Source: CAD feature listing. Evaluate the final solid. Frame: model axes, mm. Give positions to 0.01 mm unless a question says otherwise; leave off trailing zeros. Loops run counter-clockwise (first coordinate to the right, second up) from the corner with the lowest first, then second, coordinate; pieces in that order, holes last. Notation, with made-up numbers: (5.25, -20) - (39.25, -20) arc R24 cw to (39.25, 4) - close; hole circle Ø7 at (-25.5, 79). An arc over 180 degrees is marked (long way). Put each result on its own line as item: value.
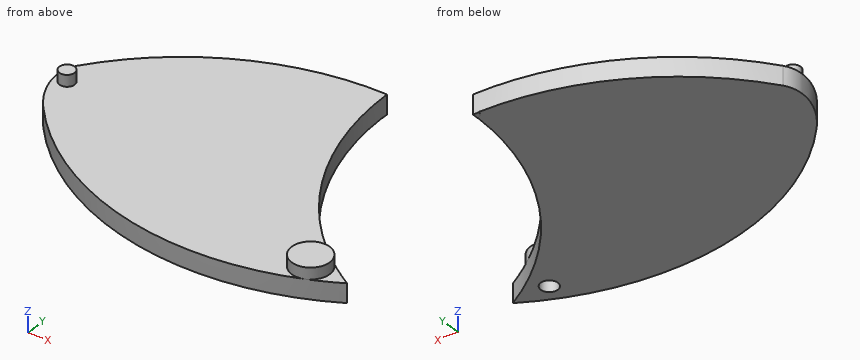
```python
from build123d import *

# Parameters (mm, degrees)
ESTRUSIONE_ESTRUSIONE1_DEPTH = 5
SCHIZZO2_R                   = 2
ESTRUSIONE_ESTRUSIONE3_DEPTH = 3
SCHIZZO3_R                   = 2.25
TAGLIO_ESTRUSIONE2_DEPTH     = 5
SCHIZZO4_R                   = 5
ESTRUSIONE_ESTRUSIONE4_DEPTH = 3
ESTRUSIONE_ESTRUSIONE5_START = -5.1
ESTRUSIONE_ESTRUSIONE5_DEPTH = 0.1


with BuildPart() as part:
    # Schizzo1 → Estrusione-Estrusione1 (new body)
    with BuildSketch(Plane.XY):
        with BuildLine():
            ThreePointArc((-62.786841774, -36.25), (-36.25, -9.713158226), (0, 0))
            ThreePointArc((0, 0), (9.713158226, -36.25), (36.25, -62.786841774))
            ThreePointArc((36.25, -62.786841774), (-18.76438077, -70.029622406), (-62.786841774, -36.25))
        make_face()
    extrude(amount=ESTRUSIONE_ESTRUSIONE1_DEPTH)

    # Schizzo2 → Estrusione-Estrusione3 (add)
    with BuildSketch(Plane.XY.offset(5)):
        with Locations(Location((-56.94020987, -36.25, 0), (0, 0, 180))):
            Circle(SCHIZZO2_R)
    extrude(amount=ESTRUSIONE_ESTRUSIONE3_DEPTH)

    # Schizzo3 → Taglio-Estrusione2 (cut)
    with BuildSketch(Plane.XY.offset(5)):
        with Locations((26.25, -62.186714819)):
            Circle(SCHIZZO3_R)
    extrude(amount=-TAGLIO_ESTRUSIONE2_DEPTH, mode=Mode.SUBTRACT)

    # Raccordo2
    # an asymmetric fillet: 16, 12 mm, written as the material it takes off along each edge
    with BuildSketch(Plane(origin=(-62.786841774, -36.25, -33.900186603), x_dir=(0.5787975585185353, -0.8154712663564442, 0), z_dir=(0, 0, 1))) as raccordo2_piece_1:
        with BuildLine():
            Bezier((13.560074641, 0), (0.046255616, -1.269344794), (-2.702341636, 6.773027618), weights=[1, 0.785330936, 1])
            ThreePointArc((-2.702341636, 6.773027618), (-1.43638067, 3.35251629), (0, 0))
            ThreePointArc((0, 0), (6.780037321, -0.317723131), (13.560074641, 0))
        make_face()
    extrude(amount=72.800373207, mode=Mode.SUBTRACT)

    # Schizzo4 → Estrusione-Estrusione4 (add)
    with BuildSketch(Plane.XY.offset(5)):
        with Locations(Location((26.25, -62.186714819, 0), (0, 0, 292.885380476))):
            Circle(SCHIZZO4_R)
    extrude(amount=ESTRUSIONE_ESTRUSIONE4_DEPTH)

    # Schizzo5 → Estrusione-Estrusione5 (add)
    with BuildSketch(Plane.XY.offset(5).offset(ESTRUSIONE_ESTRUSIONE5_START)):
        with BuildLine():
            ThreePointArc((-1.499919736, -0.015517241), (-1.04963107, -1.071575763), (0.015517241, -1.499919736))
            ThreePointArc((0.015517241, -1.499919736), (0.003879414, -0.75), (0, 0))
            ThreePointArc((0, 0), (-0.75, -0.003879414), (-1.499919736, -0.015517241))
        make_face()
    extrude(amount=ESTRUSIONE_ESTRUSIONE5_DEPTH)


solid = part.part
```
1) Material intervals for line 1 along Z through (x, y) = (9, -62); line 2 along Y through (x, z) = (28, 3.75); line 3 along X through (y, z) = (-52.5, 1.5), sorted ascending. Write a range as [from, to].
Check result:
line 1: [0, 5]
line 2: [-66.87, -63.6], [-60.77, -57.24]
line 3: [-50, 22.5]
2) Section query D-D, the plane x = -21.5. Output: boundary loops of the cut face in (y, z).
Check result:
outline: (-69.24, 0) - (-3.26, 0) - (-3.26, 5) - (-69.24, 5) - close
3) Pin query (flat end, axial travel): P1, Ø1.5, axis at x = 13.5, y = -64.5, coming from the -Z side; P2, Ø10, axis at x = -4, y = -8, coming from the +Z side; P3, Ø3, axis at x = -39.5, z = 3.5, coming from the +Y side; P4, Ø1, axis at x = -49.5, z = 6, coming from the +Y side. Return the tip coordinate at first contact, or that it passes through.
Check result:
P1: z = 0
P2: z = 5
P3: y = -10.76
P4: through
4) Section query B-B, the plane x = 26. Output: boundary loops of the cut face in (y, z).
Check result:
outline: (-67.68, 0) - (-64.42, 0) - (-64.42, 5) - (-59.95, 5) - (-59.95, 0) - (-55.62, 0) - (-55.62, 5) - (-57.19, 5) - (-57.19, 8) - (-67.18, 8) - (-67.18, 5) - (-67.68, 5) - close
5) Section query C-C, the plane y = -24. Output: boundary loops of the cut face in (x, z).
Check result:
outline: (-53.89, 0) - (4.09, 0) - (4.09, 5) - (-53.89, 5) - close
6) Section query A-A, the plane z = 6.5. Output: boundary loops of the cut face in (x, y), plus the area to 3 significant figures.
Check result:
outline: circle Ø4 at (-56.94, -36.25); circle Ø10 at (26.25, -62.19)
area: 91.1 mm²
